Build history of the part. All positions in model axes, mm. A direction names the side the tool comes from. Round coordinates to 2 decimals unless told otherwise and drop trailing zeros. Loops run counter-clockwise (first coordinate to the right, second up) from the corner with the lowest first, then second, coordinate; pieces in that order, holes last. Notation, with made-up numbers: (-22.75, 11.5) - (5.25, 11.5) arc R27 ccw to (5.25, 46.5) - close; hole circle Ø6 at (41.5, -12). An arc over 180 degrees is marked (long way). Use a Markdown table: item, result.
from build123d import *

# Parameters (mm, degrees)
SKETCH1_W           = 50
SKETCH1_H           = 85
BOSS_EXTRUDE1_DEPTH = 5
SKETCH2_R           = 1.4
CUT_EXTRUDE1_DEPTH  = 5
SKETCH3_W           = 20
SKETCH3_H           = 40
CUT_EXTRUDE2_DEPTH  = 5
FILLET3_SIZE        = 5
FILLET4_SIZE        = 5
FILLET5_SIZE        = 2.5
FILLET6_SIZE        = 2.5
SKETCH4_R           = 1.4
CUT_EXTRUDE3_DEPTH  = 5


with BuildPart() as part:
    # Sketch1 → Boss-Extrude1 (new body)
    with BuildSketch(Plane(origin=(0, 0, 0), x_dir=(1, 0, 0), z_dir=(0, 1, 0))):
        Rectangle(SKETCH1_W, SKETCH1_H)
    extrude(amount=BOSS_EXTRUDE1_DEPTH)

    # Sketch2 → Cut-Extrude1 (cut)
    with BuildSketch(Plane(origin=(0, 5, 0), x_dir=(1, 0, 0), z_dir=(0, 1, 0))):
        with Locations(Location((-14, 37.5, 0), (0, 0, 270))):
            Circle(SKETCH2_R)
        with Locations(Location((14, 37.5, 0), (0, 0, 90))):
            Circle(SKETCH2_R)
        with Locations(Location((-14, 9.5, 0), (0, 0, 270))):
            Circle(SKETCH2_R)
        with Locations(Location((14, 9.5, 0), (0, 0, 90))):
            Circle(SKETCH2_R)
    extrude(amount=-CUT_EXTRUDE1_DEPTH, mode=Mode.SUBTRACT)

    # Sketch3 → Cut-Extrude2 (cut)
    with BuildSketch(Plane(origin=(0, 5, 0), x_dir=(1, 0, 0), z_dir=(0, 1, 0))):
        with Locations((0, 22.5)):
            Rectangle(SKETCH3_W, SKETCH3_H)
    extrude(amount=-CUT_EXTRUDE2_DEPTH, mode=Mode.SUBTRACT)

    # Fillet3
    # a fillet whose section is not a circle: 5 mm, written as the material it takes off along each edge
    with BuildSketch(Plane(origin=(-25, -12.5, -42.5), x_dir=(0, 0, 1), z_dir=(0, 1, 0))) as fillet3_piece_1:
        with BuildLine():
            Bezier((FILLET3_SIZE, 0), (0, 0), (0, FILLET3_SIZE), weights=[1, 1, 1])
            Line((0, FILLET3_SIZE), (0, 0))
            Line((0, 0), (FILLET3_SIZE, 0))
        make_face()
    extrude(amount=30, mode=Mode.SUBTRACT)

    # Fillet4
    # a fillet whose section is not a circle: 5 mm, written as the material it takes off along each edge
    with BuildSketch(Plane(origin=(25, -12.5, -42.5), x_dir=(0, 0, 1), z_dir=(0, 1, 0))) as fillet4_piece_1:
        with BuildLine():
            Bezier((FILLET4_SIZE, 0), (0, 0), (0, -FILLET4_SIZE), weights=[1, 1, 1])
            Line((0, -FILLET4_SIZE), (0, 0))
            Line((0, 0), (FILLET4_SIZE, 0))
        make_face()
    extrude(amount=30, mode=Mode.SUBTRACT)

    # Fillet5
    # a fillet whose section is not a circle: 2.5 mm, written as the material it takes off along each edge
    with BuildSketch(Plane(origin=(-10, 11.25, -42.5), x_dir=(0, 0, 1), z_dir=(0, -1, 0))) as fillet5_piece_1:
        with BuildLine():
            Bezier((FILLET5_SIZE, 0), (0, 0), (0, FILLET5_SIZE), weights=[1, 1, 1])
            Line((0, FILLET5_SIZE), (0, 0))
            Line((0, 0), (FILLET5_SIZE, 0))
        make_face()
    extrude(amount=17.5, mode=Mode.SUBTRACT)

    # Fillet6
    # a fillet whose section is not a circle: 2.5 mm, written as the material it takes off along each edge
    with BuildSketch(Plane(origin=(10, 11.25, -42.5), x_dir=(0, 0, 1), z_dir=(0, -1, 0))) as fillet6_piece_1:
        with BuildLine():
            Bezier((FILLET6_SIZE, 0), (0, 0), (0, -FILLET6_SIZE), weights=[1, 1, 1])
            Line((0, -FILLET6_SIZE), (0, 0))
            Line((0, 0), (FILLET6_SIZE, 0))
        make_face()
    extrude(amount=17.5, mode=Mode.SUBTRACT)

    # Sketch4 → Cut-Extrude3 (cut)
    with BuildSketch(Plane(origin=(0, 5, 0), x_dir=(1, 0, 0), z_dir=(0, 1, 0))):
        with Locations(Location((-17, -32.5, 0), (0, 0, 270))):
            Circle(SKETCH4_R)
        with Locations(Location((17, -32.5, 0), (0, 0, 90))):
            Circle(SKETCH4_R)
        with Locations(Location((17, -12.5, 0), (0, 0, 270))):
            Circle(SKETCH4_R)
        with Locations(Location((-17, -12.5, 0), (0, 0, 90))):
            Circle(SKETCH4_R)
    extrude(amount=-CUT_EXTRUDE3_DEPTH, mode=Mode.SUBTRACT)


solid = part.part
Q1. Cut at C-C, the plane y = 1.15. Count the separate pieces of the cut face and the enclosed holes in it, plus the area to 3 significant figures.
Results found:
| item | result |
|---|---|
| separate pieces | 1 |
| enclosed holes | 8 |
| area | 3,390 mm2 |
Q2. Cut at D-D, the plane x = -9. List the corners of the cut face in (y, z).
Results found:
| item | result |
|---|---|
| outline | (0, -2.5) - (5, -2.5) - (5, 42.5) - (0, 42.5) - close |
Q3. Pull direction X, two halves, no side cores. Call faces 3 (the face through (25, 2, 3)), 4 (the face through (13.05, 2.54, -36.47)), 5 (the face through (0, 5, -1)): pulls with the +X half, pulls with the -X half, needs draft (parallel to the pull), parting line crosses it, or undercut.
Results found:
| item | result |
|---|---|
| face 3 | pulls with the +X half |
| face 4 | undercut |
| face 5 | needs draft |
Q4. Cut at B-B, the plane x = -17. List the corners of the cut face in (y, z).
Results found:
| item | result |
|---|---|
| outline | (0, -42.5) - (5, -42.5) - (5, 11.1) - (0, 11.1) - close; (0, 13.9) - (5, 13.9) - (5, 31.1) - (0, 31.1) - close; (0, 33.9) - (5, 33.9) - (5, 42.5) - (0, 42.5) - close |
Q5. Cut at A-A, the plane z = 12.5. List the corners of the cut face in (x, y), plus the area to 3 significant figures.
Results found:
| item | result |
|---|---|
| outline | (-25, 0) - (-18.4, 0) - (-18.4, 5) - (-25, 5) - close; (-15.6, 0) - (15.6, 0) - (15.6, 5) - (-15.6, 5) - close; (18.4, 0) - (25, 0) - (25, 5) - (18.4, 5) - close |
| area | 222 mm2 |
Q6. Which spindle directions (+Z, -Z, +X, -X, +Y, -Y) get a long thin tool onto all of the face, cutting with end or side? Do faces 1 (the face through (-10, 3, -21)), 2 (the face through (17.06, 2.54, 11.1)). Say none if no direction does.
Results found:
| item | result |
|---|---|
| face 1 | -Z, +Y, -Y |
| face 2 | +Y, -Y |
Q7. Probe line 1 (X direction, y = 1.8, z = 32.5); line 2 (X direction, y = 3.6, z = -37.5); line 3 (Z direction, x = 16, y = 2.35). List the from-to ranges inside material, lowest first.
Results found:
| item | result |
|---|---|
| line 1 | x = -25 to -18.4, -15.6 to 15.6, 18.4 to 25 |
| line 2 | x = -25 to -15.4, -12.6 to -10, 10 to 12.6, 15.4 to 25 |
| line 3 | z = -42.5 to 11.52, 13.48 to 31.52, 33.48 to 42.5 |
Q8. Drop a flat-ended pin along its axis: pin 1 (2 mm diameter, centred on x = 17, z = 12.5, fed in from +Y). Give the stop position or say it passes through.
Results found:
| item | result |
|---|---|
| pin 1 | passes through |
